Build history of the part. All positions in model axes, mm. Give positions to 0.01 mm unless a question says otherwise; leave off trailing zeros. Order: outer loops, then holes, each group sorted by start corner. A loop starts at its lowest first (then second) coordinate and runs counter-clockwise, first axis right, second up. Notation, with made-up numbers: (-23, 55) -> (-9, 55) arc R23 ccw to (-9, 85) -> close; hole circle Ø7 at (44, -6.5). An arc over 180 degrees is marked (long way). One line per question, with ' | ' between items. Start each with the question number.
(1) Pin check, flat tips, straight feed: pin 1 Ø4 at (x, y) = (-6, 21.5) entering from +Z; pin 2 Ø6 at (x, y) = (-35.5, 24) entering from +Z; pin 3 Ø5 at (x, z) = (2.5, -20) entering from -Y. Stop position of each tip, or through.
(2) Cut at B-B (z = 22). Give the cut face in (x, y).
(3) Cut at A-A (x = -2). Give the cut face in (y, z), then the cut area to 3 significant figures.
(4) Drill centre lines: L1, parallel to Z at x = -4.5, y = 47; L2, parallel to Z at x = 8.5, y = 31; L3, parallel to Y at x = -12.5, z = -17.5. Where is each one in solid material? Low to high. Write a range as from..to.
(5) Cut at C-C (y = 35.5). Give the cut face in (x, z), then the cut area to 3 significant figures.
from build123d import *

# Parameters (mm, degrees)
SKETCH1_W           = 100
SKETCH1_H           = 60
BOSS_EXTRUDE1_DEPTH = 60
CUT_EXTRUDE1_DEPTH  = 100


with BuildPart() as part:
    # Sketch1 → Boss-Extrude1 (new body)
    with BuildSketch(Plane(origin=(0, 0, 0), x_dir=(1, 0, 0), z_dir=(0, 1, 0))):
        Rectangle(SKETCH1_W, SKETCH1_H)
    extrude(amount=BOSS_EXTRUDE1_DEPTH)

    # Sketch2 → Cut-Extrude1 (cut)
    with BuildSketch(Plane(origin=(50, 0, 0), x_dir=(0, 0, -1), z_dir=(1, 0, 0))):
        Polygon((-30, 60), (-30, 16.698729811), (-5, 60), align=None)
        Polygon((30, 0), (30, 23.873553173), (16.216597649, 0), align=None)
        Polygon((23.232724571, 60), (30, 60), (30, 52.540618633), align=None)
    extrude(amount=-CUT_EXTRUDE1_DEPTH, mode=Mode.SUBTRACT)


solid = part.part
Result set:
1) pin 1: stops at z = 28.38 | pin 2: stops at z = 27.52 | pin 3: stops at y = 2.22
2) outline: (-50, 0) -> (50, 0) -> (50, 30.56) -> (-50, 30.56) -> close
3) outline: (0, -16.22) -> (23.87, -30) -> (52.54, -30) -> (60, -23.23) -> (60, 5) -> (16.7, 30) -> (0, 30) -> close | area: 2,870 mm2
4) L1: z = -30..12.51 | L2: z = -30..21.74 | L3: y = 2.22..60
5) outline: (-50, -30) -> (50, -30) -> (50, 19.15) -> (-50, 19.15) -> close | area: 4,910 mm2
